Read the model definition and answer for the solid it produces. Units are mm, in the model's axes. Face numbers are marked on the shaded views. A direction names the side the tool comes from. Give positions to 0.01 mm unless a question says otherwise; leave off trailing zeros. Order: outer loops, then holes, each group sorted by start corner. A loop starts at its lowest first (then second) coordinate and runs counter-clockwise, first axis right, second up. Notation, with made-up numbers: (52, 39) -> (76, 39) arc R20 cw to (76, 59) -> close; hole circle Ø1 at (61.5, 83.5). An arc over 180 degrees is marked (long way). Answer as CSV lines item,"result". Start each with the question number.
1) The mould has two halves that part along X. Classify the marked faces 1, 2 and 3: +X half, -X half, draft (parallel to the pull), parting line (faces both ways), or undercut.
2) Straight lines are drawn through the part: L1, parallel to X at y = -41, z = 0.25; L2, parallel to X at y = -39.5, z = 0; L3, parallel to Y at x = -31, z = 1. For each, find the intervals that lie inside material, in ascending order. Write a range as from..to.
3) Find section B-B (y = -32). Determine the outline of the cut face in (x, z), and give its area (3 significant figures).
4) Find section D-D (x = -31.75). Determine the outline of the cut face in (y, z), and give its area (4 significant figures).
5) Find section C-C (y = -51.5). Determine the outline of the cut face in (x, z).
6) Flat-ended cylindrical pins translate along their axes: pin 1 Ø9 at (x, z) = (-9.5, -2.5) entering from +Y; pin 2 Ø4 at (y, z) = (-50.5, 4.5) entering from +X; pin 3 Ø5.5 at (x, y) = (10.5, 1.5) entering from -Z; pin 4 Ø4 at (y, z) = (-46, -6) entering from -X. Find the tip coordinate at first contact, or state that the pin passes through.
7) For the marked faces 4, 5, 6, 7 and 8, determine the directions among +Z, -Z, +X, -X, +Y, -Y from which every point of the face is accessible in a straight line to the end or side of a thin tool.
8) Find section A-A (x = -13). Determine the outline of the cut face in (y, z).
```python
from build123d import *

# Parameters (mm, degrees)
EXTRUDE_1_DEPTH = 9.25
SKETCH_2_R      = 7.5
EXTRUDE_2_DEPTH = 15
SKETCH_3_R      = 4
EXTRUDE_3_DEPTH = 20
SKETCH_4_R      = 2.5
EXTRUDE_4_DEPTH = 15
EXTRUDE_5_DEPTH = 5
SKETCH_6_R      = 1.5
EXTRUDE_6_DEPTH = 6


with BuildPart() as part:
    # 草图1 → 凸台-拉伸1 (new, symmetric)
    with BuildSketch(Plane.XY):
        Polygon((36, 0), (-36, 0), (-36, -27), (-24, -27), (-11, -40), (11, -40), (24, -27), (36, -27), align=None)
    extrude(amount=EXTRUDE_1_DEPTH, both=True)

    # 草图2 → 凸台-拉伸2 (add)
    with BuildSketch(Plane.XZ.offset(40)):
        with Locations(Location((0, 0, 0), (0, 0, 90))):
            Circle(SKETCH_2_R)
    extrude(amount=EXTRUDE_2_DEPTH)

    # 草图3 → 凸台-拉伸3 (add)
    with BuildSketch(Plane.XZ.offset(55)):
        with Locations(Location((0, 0, 0), (0, 0, 270))):
            Circle(SKETCH_3_R)
    extrude(amount=EXTRUDE_3_DEPTH)

    # 草图4 → 凸台-拉伸4 (add)
    with BuildSketch(Plane.XZ.offset(27)):
        with Locations(Location((-31.75, 0, 0), (0, 0, 90))):
            Circle(SKETCH_4_R)
        with Locations(Location((31.75, 0, 0), (0, 0, 90))):
            Circle(SKETCH_4_R)
    extrude(amount=EXTRUDE_4_DEPTH)

    # 草图5 → 凸台-拉伸5 (add)
    with BuildSketch(Plane(origin=(0, 0, 0), x_dir=(1, 0, 0), z_dir=(0, 1, 0))):
        Polygon((-27, 4), (27, 4), (25.5, -4), (-25.5, -4), align=None)
    extrude(amount=EXTRUDE_5_DEPTH)

    # 草图6 → 凸台-拉伸6 (add)
    with BuildSketch(Plane(origin=(0, 0, 0), x_dir=(1, 0, 0), z_dir=(0, 1, 0))):
        with Locations((-31.75, 0)):
            Circle(SKETCH_6_R)
        with Locations((31.75, 0)):
            Circle(SKETCH_6_R)
    extrude(amount=EXTRUDE_6_DEPTH)


solid = part.part
```
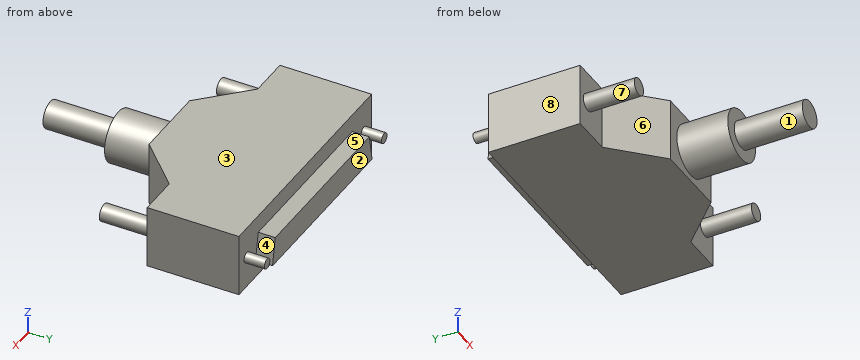
Findings below:
1,face 1,"parting line"
1,face 2,"undercut"
1,face 3,"draft"
2,L1,"-34.24..-29.26, -7.5..7.5, 29.26..34.24"
2,L2,"-34.25..-29.25, -11.5..11.5, 29.25..34.25"
2,L3,"-42..6"
3,outline,"circle Ø5 at (-31.75, 0); (-19, -9.25) -> (19, -9.25) -> (19, 9.25) -> (-19, 9.25) -> close; circle Ø5 at (31.75, 0)"
3,area,"742 mm²"
4,outline,"(-42, -2.5) -> (-27, -2.5) -> (-27, -9.25) -> (0, -9.25) -> (0, -1.5) -> (6, -1.5) -> (6, 1.5) -> (0, 1.5) -> (0, 9.25) -> (-27, 9.25) -> (-27, 2.5) -> (-42, 2.5) -> close"
4,area,"592.5 mm²"
5,outline,"circle Ø15 at (0, 0)"
6,pin 1,"y = 5"
6,pin 2,"x = 7.07"
6,pin 3,"z = -9.25"
6,pin 4,"x = -6.34"
7,face 4,"+Z, +Y"
7,face 5,"+Z, +X, -X, +Y"
7,face 6,"+Z, -Z, -Y"
7,face 7,"-Y"
7,face 8,"+Z, -Z, -X, +Y, -Y"
8,outline,"(-38, -9.25) -> (0, -9.25) -> (0, -4) -> (5, -4) -> (5, 4) -> (0, 4) -> (0, 9.25) -> (-38, 9.25) -> close"
